from build123d import *

# Parameters (mm, degrees)
F0_R          = 37.5
F1_DEPTH      = 84
F1_DEPTH_BACK = 84
F2_DEPTH      = 89
F2_DEPTH_BACK = 89
F3_W          = 76
F3_H          = 131.6358613752
F3_R          = 37.5
F4_DEPTH      = 650


with BuildPart() as f1:
    # F0 (on Front) → F1 (new body, two sides)
    with BuildSketch(Plane.XZ) as f1_sk:
        with BuildLine():
            Line((-65.8179306876, 38), (-65.8179306876, -38))
            ThreePointArc((-65.8179306876, -38), (-53.7401153702, -53.7401153702), (-38, -65.8179306876))
            Line((-38, -65.8179306876), (38, -65.8179306876))
            ThreePointArc((38, -65.8179306876), (53.7401153702, -53.7401153702), (65.8179306876, -38))
            Line((65.8179306876, -38), (65.8179306876, 38))
            ThreePointArc((65.8179306876, 38), (53.7401153702, 53.7401153702), (38, 65.8179306876))
            Line((38, 65.8179306876), (-38, 65.8179306876))
            ThreePointArc((-38, 65.8179306876), (-53.7401153702, 53.7401153702), (-65.8179306876, 38))
        make_face()
        Circle(F0_R, mode=Mode.SUBTRACT)
        Circle(F0_R)
    extrude(amount=F1_DEPTH)
    extrude(f1_sk.sketch, amount=-F1_DEPTH_BACK)

    # F0 (on Front) → F2 (join, two sides)
    with BuildSketch(Plane.XZ) as f2_sk:
        Circle(F0_R)
    extrude(amount=F2_DEPTH)
    extrude(f2_sk.sketch, amount=-F2_DEPTH_BACK)

    # F3 (on face) → F4 (join)
    with BuildSketch(Plane(origin=(0, 0, -65.8179306876), x_dir=(1, 0, 0), z_dir=(0, 0, -1))):
        Rectangle(F3_W, F3_H)
        Circle(F3_R, mode=Mode.SUBTRACT)
        Circle(F3_R)
        with BuildLine():
            Line((-65.8179306876, 38), (-65.8179306876, -38))
            ThreePointArc((-65.8179306876, -38), (-53.7401153702, -53.7401153702), (-38, -65.8179306876))
            Line((-38, -65.8179306876), (-38, 65.8179306876))
            ThreePointArc((-38, 65.8179306876), (-53.7401153702, 53.7401153702), (-65.8179306876, 38))
        make_face()
        with BuildLine():
            Line((38, 65.8179306876), (38, -65.8179306876))
            ThreePointArc((38, -65.8179306876), (53.7401153702, -53.7401153702), (65.8179306876, -38))
            Line((65.8179306876, -38), (65.8179306876, 38))
            ThreePointArc((65.8179306876, 38), (53.7401153702, 53.7401153702), (38, 65.8179306876))
        make_face()
    extrude(amount=F4_DEPTH)


solid = f1.part
For this review, take the finished solid that the model builds, in its own axes (mm). A direction names the side the tool comes from. Round coordinates to 2 decimals unless told otherwise and drop trailing zeros. Write each loop counter-clockwise with the first axis right and the second up, starting at its lowest first coordinate (ties: lowest second). Pieces come first, ordered by that corner, then holes. Notation, with made-up numbers: (-9, 19) -> (44, 19) arc R22 ccw to (44, 40) -> close; hole circle Ø4 at (-38, 22.5). An arc over 180 degrees is marked (long way). Put each result on its own line as item: value.
Q1. Consider section A-A on x = 0. State the section outline as (y, z) points, and give its area (3 significant figures).
Determined:
outline: (-89, -37.5) -> (-84, -37.5) -> (-84, -65.82) -> (-65.82, -65.82) -> (-65.82, -715.82) -> (65.82, -715.82) -> (65.82, -65.82) -> (84, -65.82) -> (84, -37.5) -> (89, -37.5) -> (89, 37.5) -> (84, 37.5) -> (84, 65.82) -> (-84, 65.82) -> (-84, 37.5) -> (-89, 37.5) -> close
area: 108,000 mm^2
Q2. Consider section C-C on x = 45. State the section outline as (y, z) points.
Determined:
outline: (-84, -61.25) -> (84, -61.25) -> (84, 61.25) -> (-84, 61.25) -> close; (-61.25, -715.82) -> (61.25, -715.82) -> (61.25, -65.82) -> (-61.25, -65.82) -> close
Q3. To check wall thickness, follow L1, parallel to Z at x = -3, y = 71.5; L2, parallel to Y at x = 5, z = -41. State the ranges of each line that lie inside material, in increasing order. Write a range as [from, to].
Determined:
L1: z = [-65.82, 65.82]
L2: y = [-84, 84]
Q4. Clearance check with flat-ended pins moving along their axes: pin 1 Ø12 at (x, z) = (-4.5, -361.5) entering from -Y; pin 2 Ø1.5 at (y, z) = (-39, -129) entering from +X; pin 3 Ø9 at (x, y) = (11.5, -72.5) entering from -Z. State where each tip first meets the part, or that it passes through.
Determined:
pin 1: stops at y = -65.82
pin 2: stops at x = 65.67
pin 3: stops at z = -65.82
Q5. Machinability: for faces 1 (the flat face through (-30, 84, -28)), 2 (the cylindrical face through (-53.94, 53.54, -386.27)), 3 (the cylindrical face through (-53.54, -53.94, -386.27)), 4 (the flat face through (-1, 75, -65.818)), which of the approach directions +Z, -Z, +X, -X, +Y, -Y give a long, thin tool a straight path to every point of the face, cutting with its end or side? Answer none if there is none.
Determined:
face 1: +Y
face 2: -Z, -X, +Y
face 3: -Z, -X, -Y
face 4: -Z, +X, -X, +Y
Q6. Consider section D-D on y = 47. State the section outline as (x, z) points.
Determined:
outline: (-65.82, -38) arc R76 ccw to (-38, -65.82) -> (-59.72, -65.82) -> (-59.72, -715.82) -> (59.72, -715.82) -> (59.72, -65.82) -> (38, -65.82) arc R76 ccw to (65.82, -38) -> (65.82, 38) arc R76 ccw to (38, 65.82) -> (-38, 65.82) arc R76 ccw to (-65.82, 38) -> close
Q7. Consider section B-B on z = -601.5. State the section outline as (x, y) points, and give its area (3 significant figures).
Determined:
outline: (-65.82, -38) arc R76 ccw to (-38, -65.82) -> (38, -65.82) arc R76 ccw to (65.82, -38) -> (65.82, 38) arc R76 ccw to (38, 65.82) -> (-38, 65.82) arc R76 ccw to (-65.82, 38) -> close
area: 16,100 mm^2
Q8. The part is to be moulded in two halves that separate along Z. For faces 5 (the cylindrical face through (53.94, -53.54, -386.27)), 6 (the cylindrical face through (-4.88, -86.46, 37.18)), 7 (the flat face through (-52, -1, -65.818)), say which applies: released by +Z, released by -Z, zero draft, split by the parting line, or undercut.
Determined:
face 5: zero draft
face 6: split by the parting line
face 7: undercut
